Work out the finished part from the listing and answer in its coordinate system (mm). Face numbers are marked on the shaded views. A direction names the side the tool comes from. Round coordinates to 2 decimals unless told otherwise and drop trailing zeros. Write each loop counter-clockwise with the first axis right and the second up, starting at its lowest first coordinate (ties: lowest second). Pieces come first, ordered by that corner, then holes.
1. Determine the mould class of the marked faces 1, 2 and 3 for opening direction X: pulls with the +X half, pulls with the -X half, needs draft (parallel to the pull), parting line crosses it, or undercut.
2. Find section C-C (x = -96). Write down the section's boundary in (y, z), and give its area (3 significant figures).
3. A tool of negligible diameter and unlimited length cuts with its end or side. For the marked faces 4 and 5, from which of +Z, -Z, +X, -X, +Y, -Y can it reach the whole face along a straight path? Write none if from no direction.
4. Find section B-B (y = 21). Write down the section's boundary in (x, z).
5. Find section A-A (z = 47.5). Write down the section's boundary in (x, y), and give its area (3 significant figures).
6. Straight lines are drawn through the part: probe 1 along X at (y, z) = (31.5, 76); probe 2 along Y at (x, z) = (-49.5, 95.5); probe 3 along X at (y, z) = (1.5, 139). For each, find the intervals that lie inside material, in ascending order.
7. Flat-ended cylindrical pins translate along their axes: pin 1 Ø4 at (y, z) = (5.16, 149.22) entering from +X; pin 2 Ø2 at (x, z) = (-63.5, 88.5) entering from +Y. Find the tip coordinate at first contact, or state that the pin passes through.
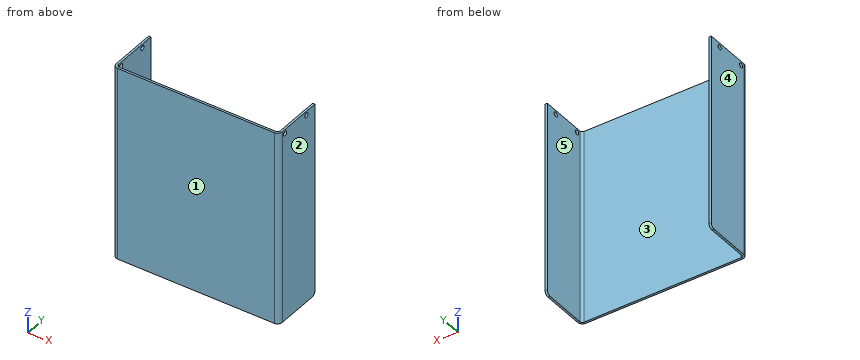
```python
from build123d import *

# Parameters (mm, degrees)
F1_DEPTH = 152.4
F2_R     = 1.98374
F3_R     = 3.69316
F4_R     = 1.8288
F5_DEPTH = 130.41884
F6_R     = 3.175


with BuildPart() as f1:
    # F0 (on Top) → F1 (new body)
    with BuildSketch(Plane.XY):
        Polygon((0, 38.8047992), (0, 0), (-127, 0), (-127, 38.8047992), (-128.70942, 38.8047992), (-128.70942, -1.70942), (1.70942, -1.70942), (1.70942, 38.8047992), align=None)
    extrude(amount=F1_DEPTH)

    # F2
    f2_edges = [f1.edges().sort_by_distance(p)[0] for p in [
        (0, 0, 76.2),
        (-127, 0, 76.2),
    ]]
    fillet(f2_edges, radius=F2_R)

    # F3
    f3_edges = [f1.edges().sort_by_distance(p)[0] for p in [
        (1.70942, -1.70942, 76.2),
        (-128.70942, -1.70942, 76.2),
    ]]
    fillet(f3_edges, radius=F3_R)

    # F4 (on face) → F5 (cut, through all)
    with BuildSketch(Plane(origin=(-128.70942, 0, 0), x_dir=(0, -1, 0), z_dir=(-1, 0, 0))):
        with Locations((-29.2797992, 149.225)):
            Circle(F4_R)
        with Locations((-5.15874, 149.225)):
            Circle(F4_R)
    extrude(amount=-F5_DEPTH, mode=Mode.SUBTRACT)

    # F6
    f6_edges = [f1.edges().sort_by_distance(p)[0] for p in [
        (0.85471, 38.804799, 0),
        (-127.85471, 38.804799, 0),
    ]]
    fillet(f6_edges, radius=F6_R)


solid = f1.part
```
Worked answers:
1. face 1: needs draft
1. face 2: pulls with the +X half
1. face 3: undercut
2. outline: (-1.71, 0) - (0, 0) - (0, 152.4) - (-1.71, 152.4) - close
2. area: 261 mm2
3. face 4: +Z, -Z, -X, +Y, -Y
3. face 5: +Z, -Z, +Y
4. outline: (-128.71, 0) - (-127, 0) - (-127, 152.4) - (-128.71, 152.4) - close; (0, 0) - (1.71, 0) - (1.71, 152.4) - (0, 152.4) - close
5. outline: (-128.71, 1.98) arc R3.69 ccw to (-125.02, -1.71) - (-1.98, -1.71) arc R3.69 ccw to (1.71, 1.98) - (1.71, 38.8) - (0, 38.8) - (0, 1.98) arc R1.98 cw to (-1.98, 0) - (-125.02, 0) arc R1.98 cw to (-127, 1.98) - (-127, 38.8) - (-128.71, 38.8) - close
5. area: 351 mm2
6. probe 1: x = -128.71 to -127, 0 to 1.71
6. probe 2: y = -1.71 to 0
6. probe 3: x = -128.68 to -126.94, -0.06 to 1.68
7. pin 1: stops at x = 1.71
7. pin 2: stops at y = 0
